Can you work these out from the model? Positions are in its coordinate system, mm. A direction names the side the tool comes from. Coordinates: 2 decimals unless noted, no trailing zeros. Write each loop counter-clockwise with the first axis right and the second up, starting at its lowest first coordinate (ties: lowest second). Pieces come first, ordered by that corner, then holes. Notation, with made-up numbers: M 72,-10.75 L 131,-10.75 A27 ccw 131,25.25 Z; hole C 20.5,-5 d8. An arc over 180 degrees is marked long. Answer as a JSON object with one key per item and string values. Group by question number.
from build123d import *

# Parameters (mm, degrees)
F1_DEPTH = 228.6
F2_DEPTH = 152.4
F3_W     = 457.2
F3_H     = 6.35
F4_DEPTH = 762


with BuildPart() as f1:
    # F0 (on Front) → F1 (new body, symmetric)
    with BuildSketch(Plane.XZ):
        with BuildLine():
            Line((739.566909, 0), (762, 0))
            ThreePointArc((762, 0), (0, 204.177285), (-762, 0))
            Line((-762, 0), (-739.566909, 0))
            ThreePointArc((-739.566909, 0), (0, 191.477285), (739.566909, 0))
        make_face()
    extrude(amount=F1_DEPTH, both=True)

    # F0 (on Front) → F2 (cut, symmetric)
    with BuildSketch(Plane.XZ):
        with BuildLine():
            Line((739.566909, 0), (762, 0))
            ThreePointArc((762, 0), (0, 204.177285), (-762, 0))
            Line((-762, 0), (-739.566909, 0))
            ThreePointArc((-739.566909, 0), (0, 191.477285), (739.566909, 0))
        make_face()
    extrude(amount=F2_DEPTH, both=True, mode=Mode.SUBTRACT)

    # F3 (on Right) → F4 (join, symmetric)
    with BuildSketch(Plane.YZ):
        with Locations((0, -3.175)):
            Rectangle(F3_W, F3_H)
    extrude(amount=F4_DEPTH, both=True)


solid = f1.part
Q1. On a 3-axis mill with a long thin cutter (end or side, diameter ignored), from which of +Z, -Z, +X, -X, +Y, -Y can I reach the whole of each face in a straight line? I mean faces 4 (the cylindrical face through (11.171, 189.967, 204.136)), 5 (the flat face through (-4, 152.4, 193)). Say none if no direction works.
Q2. We'd pull the mould along X, two halves only. Please class faces 1 (the flat face through (11, -3, 0)), 2 (the cylindrical face through (11.171, -191.033, 204.136)), 3 (the flat face through (4, 228.6, -3)): pulls with the +X half, pulls with the -X half, needs draft (parallel to the pull), parting line crosses it, or undercut.
Q3. If we section it at B-B on y = 174: List the corners of the cut face in (x, z) for me.
Q4. If we section it at C-C on x = -155: List the corners of the cut face in (y, z) for me, and give its area (3 significant figures).
Q5. Please list where these lines run through material, in increasing order: L1, parallel to Y at x = -469, z = 118; L2, parallel to Z at x = 693.5, y = -14; L3, parallel to Z at x = -283.5, y = 166.
Q6. Will these pins go through, and if not, where does the flat tip stop? pin 1 (10 mm diameter, centred on y = 151, z = 19.5, fed in from -X); pin 2 (1.5 mm diameter, centred on y = 167.5, z = 59.5, fed in from +X).
Q7. If we section it at D-D on z = 139: List the corners of the cut face in (x, y) for me.
Reply:
{
 "1": {"face 4": "+Z, +Y, -Y", "face 5": "+Z, +X, -X"},
 "2": {"face 1": "undercut", "face 2": "parting line crosses it", "face 3": "needs draft"},
 "3": {"outline": "M -762,-6.35 L 762,-6.35 L 762,0 A1524 ccw -762,0 Z; hole M -739.57,0 L 739.57,0 A1524 ccw Z"},
 "4": {"outline": "M -228.6,-6.35 L 228.6,-6.35 L 228.6,0 L -228.6,0 Z; M -228.6,183.57 L -152.4,183.57 L -152.4,196.27 L -228.6,196.27 Z; M 152.4,183.57 L 228.6,183.57 L 228.6,196.27 L 152.4,196.27 Z", "area": "4,840 mm^2"},
 "5": {"L1": "-228.6 to -152.4, 152.4 to 228.6", "L2": "-6.35 to 0", "L3": "-6.35 to 0, 164.88 to 177.58"},
 "6": {"pin 1": "x = -735.95", "pin 2": "x = 649.7"},
 "7": {"outline": "M -440.92,-228.6 L -396.48,-228.6 L -396.48,-152.4 L -440.92,-152.4 Z; M -440.92,152.4 L -396.48,152.4 L -396.48,228.6 L -440.92,228.6 Z; M 396.48,-228.6 L 440.92,-228.6 L 440.92,-152.4 L 396.48,-152.4 Z; M 396.48,152.4 L 440.92,152.4 L 440.92,228.6 L 396.48,228.6 Z"}
}
